Can you work these out from the drawing? Everything is in mm from the part's minimum corner. A direction names the side the tool comes from. Give positions to 0.01 mm unless a question says otherwise; leave off trailing zeros. Order: outer loops, then holes, each group sorted by start corner. A loop starts at its lowest first (then second) coordinate and runs counter-clockwise, first axis right, second up. Notation, with made-up numbers: (-36, 62) - (13, 62) arc R19 cw to (13, 82) - close; hole circle Ø3 at (-15, 86.25). An arc over 180 degrees is marked (long way). Answer as a JSON object with one key per item and string values.
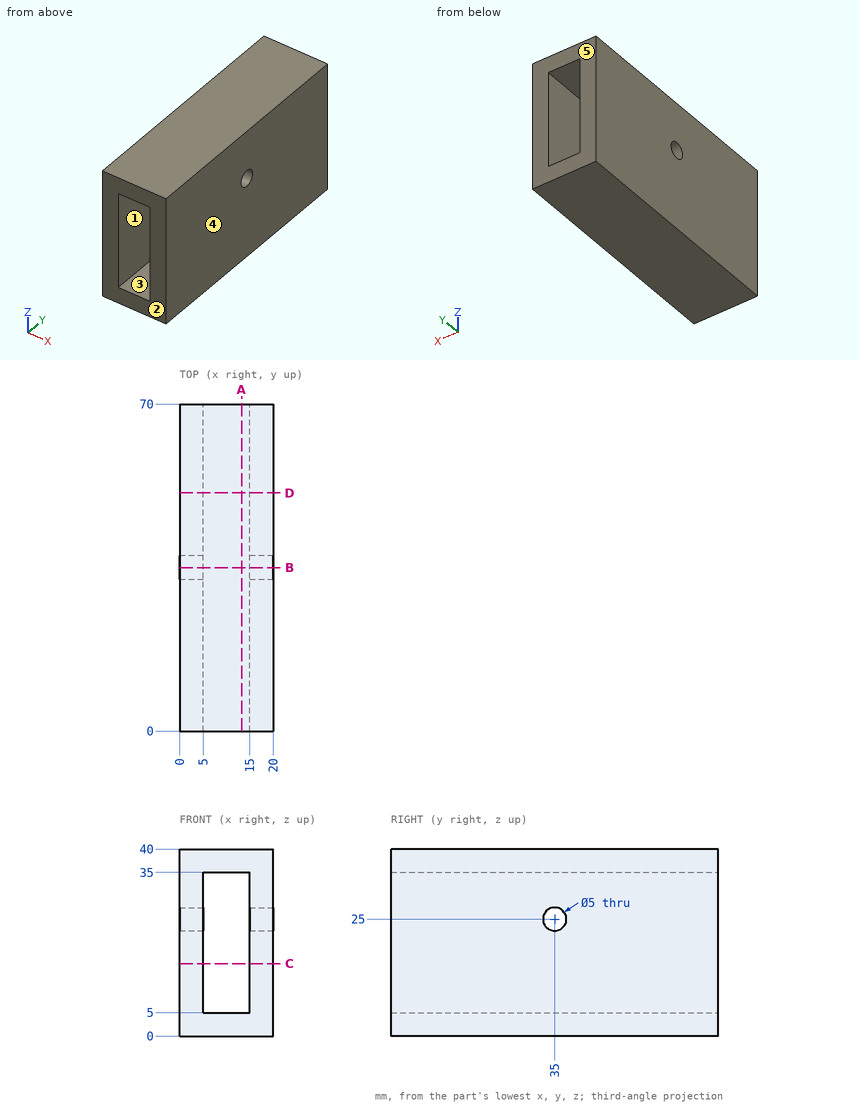
Q1. I need wall thicknesses on L1, parallel to X at y = 64.5, z = 33; L2, parallel to Z at x = 1.3, y = 35; L3, parallel to Z at x = 14, y = 45. Which ranges of each line are inside material? Lowest first, please.
Recorded:
{"L1": "x = 0 to 5, 15 to 20", "L2": "z = 0 to 22.5, 27.5 to 40", "L3": "z = 0 to 5, 35 to 40"}
Q2. If we section it at A-A, the plane x = 13.25: Please give me the cut outline in (y, z).
Recorded:
{"outline": "(0, 0) - (70, 0) - (70, 5) - (0, 5) - close; (0, 35) - (70, 35) - (70, 40) - (0, 40) - close"}
Q3. If we section it at C-C, the plane z = 15.5: Please give me the cut outline in (x, y).
Recorded:
{"outline": "(0, 0) - (5, 0) - (5, 70) - (0, 70) - close; (15, 0) - (20, 0) - (20, 70) - (15, 70) - close"}
Q4. Which directions (+Z, -Z, +X, -X, +Y, -Y) give clear straight access to the entire face, cutting with the end or side of a thin tool? Please do the marked faces 1 and 2.
Recorded:
{"face 1": "+Y, -Y", "face 2": "+Z, -Z, +X, -X, -Y"}
Q5. We'd pull the mould along X, two halves only. Please class the marked faces 3, 4 and 5: released by +X, released by -X, zero draft, split by the parting line, or undercut.
Recorded:
{"face 3": "undercut", "face 4": "released by +X", "face 5": "zero draft"}
Q6. If we section it at B-B, the plane y = 35: Please give me the cut outline in (x, z), then the cut area to 3 significant figures.
Recorded:
{"outline": "(0, 0) - (20, 0) - (20, 22.5) - (15, 22.5) - (15, 5) - (5, 5) - (5, 22.5) - (0, 22.5) - close; (0, 27.5) - (5, 27.5) - (5, 35) - (15, 35) - (15, 27.5) - (20, 27.5) - (20, 40) - (0, 40) - close", "area": "450 mm^2"}
Q7. If we section it at D-D, the plane y = 51: Please give me the cut outline in (x, z).
Recorded:
{"outline": "(0, 0) - (20, 0) - (20, 40) - (0, 40) - close; hole (5, 5) - (15, 5) - (15, 35) - (5, 35) - close"}
